Source: CAD feature listing. Evaluate the final solid. Frame: model axes, mm. Face numbers are marked on the shaded views. A direction names the side the tool comes from. Coordinates: 2 decimals unless noted, no trailing zeros. Loops run counter-clockwise (first coordinate to the right, second up) from the corner with the lowest first, then second, coordinate; pieces in that order, holes last.
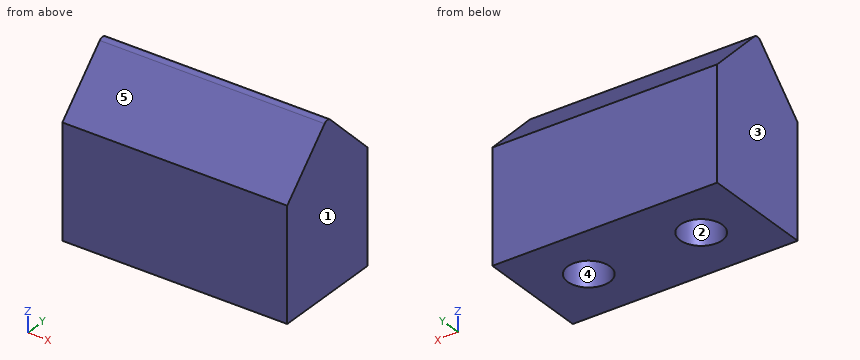
from build123d import *

# Parameters (mm, degrees)
F0_W     = 12.7
F0_H     = 12.7
F1_DEPTH = 25.4
F3_D     = 4.7625
F3_DEPTH = 9.525
F3_TIP   = 1.4307993491
F4_R     = 0.635


with BuildPart() as f1:
    # F0 (on Right) → F1 (new body)
    with BuildSketch(Plane.YZ):
        with Locations((6.35, 6.35)):
            Rectangle(F0_W, F0_H)
        Polygon((6.35, 19.05), (0, 12.7), (12.7, 12.7), align=None)
    extrude(amount=F1_DEPTH)

    # F3
    with Locations(Plane(origin=(0, 0, 0), x_dir=(1, 0, 0), z_dir=(0, 0, -1))):
        with Locations((6.35, -6.35), (19.05, -6.35)):
            Hole(F3_D / 2, depth=F3_DEPTH)
            with Locations((0, 0, -(F3_DEPTH + F3_TIP / 2))):  # 118° drill point
                Cone(0, F3_D / 2, F3_TIP, mode=Mode.SUBTRACT)

    # F4
    f4_edges = [f1.edges().sort_by_distance(p)[0] for p in [
        (12.7, 6.35, 19.05),
    ]]
    fillet(f4_edges, radius=F4_R)


solid = f1.part
Q1. Section C-C, the plane y = 2. Return the cut outline in (x, z).
Q2. Draft query along X for the marked faces 1, 2 and 3. Return one class per face: +X half, -X half, draft (parallel to the pull), parting line (faces both ways), or undercut.
Q3. Access query for the marked faces 4 and 5. Directions: +Z, -Z, +X, -X, +Y, -Y. A direction counts if a zero-diameter tool reaches every point of the face in a straight line with its end or side. Return the directions, or none.
Q4. Contact query for a flat-ended pin moving along its axis: pin 1 Ø6 at (x, y) = (8.5, 11.5) entering from +Z. Output: stop coordinate, or through.
Q5. Section A-A, the plane z = 6. Return the cut outline in (x, y), plus the area to 3 significant figures.
Q6. Section B-B, the plane x = 23.5. Return the cut outline in (y, z) (3 decimals).
Q7. Section D-D, the plane z = 15. Return the cut outline in (x, y), plus the area to 3 significant figures.
Q8. Line query: line 1 along Y through (x, z) = (19.05, 5.5); line 2 along X through (y, z) = (8.5, 9.25); line 3 along Y through (x, z) = (5.5, 2.75). Output: solid intervals per line, ascending.
Derived:
1. outline: (0, 0) - (25.4, 0) - (25.4, 14.7) - (0, 14.7) - close
2. face 1: +X half
2. face 2: undercut
2. face 3: -X half
3. face 4: -Z
3. face 5: +Z, +X, -X, -Y
4. pin 1: stops at z = 16.9
5. outline: (0, 0) - (25.4, 0) - (25.4, 12.7) - (0, 12.7) - close; hole circle Ø4.76 at (6.35, 6.35); hole circle Ø4.76 at (19.05, 6.35)
5. area: 287 mm2
6. outline: (0, 0) - (12.7, 0) - (12.7, 12.7) - (6.799, 18.601) arc R0.635 ccw to (5.901, 18.601) - (0, 12.7) - close
7. outline: (0, 2.3) - (25.4, 2.3) - (25.4, 10.4) - (0, 10.4) - close
7. area: 206 mm2
8. line 1: y = 0 to 3.97, 8.73 to 12.7
8. line 2: x = 0 to 5.33, 7.37 to 18.03, 20.07 to 25.4
8. line 3: y = 0 to 4.13, 8.57 to 12.7
